Source: CAD feature listing. Evaluate the final solid. Frame: model axes, mm. A direction names the side the tool comes from. Coordinates: 2 decimals unless noted, no trailing zeros. Write each loop counter-clockwise with the first axis right and the second up, starting at its lowest first coordinate (ties: lowest second). Pieces come first, ordered by that corner, then holes. Notation, with made-up numbers: M -27,31.25 L 21,31.25 A22 ccw 21,43.25 Z; hole C 39,34.25 d8. An arc over 180 degrees is marked long. One line per item, written item: value. Start each with the question number.
Item 1: Cut plane A-A, the plane x = 0. Output: boundary loops of the cut face in (y, z), then the cut area to 3 significant figures.
Item 2: Cut plane C-C, the plane z = -10. Output: boundary loops of the cut face in (x, y).
Item 3: Cut plane D-D, the plane z = -14.25. Output: boundary loops of the cut face in (x, y), then the cut area to 3 significant figures.
Item 4: Set-up query: faces 1 (the flat face through (-2, -35, -5)), 2 (the flat face through (10, -28, 4)), 3 (the flat face through (5, 5, 7)). Return all of +Z, -Z, +X, -X, +Y, -Y with unobstructed straight access to the full face (end or side cutting, diameter ignored); none if empty.
Item 5: Cut plane B-B, the plane z = 5. Output: boundary loops of the cut face in (x, y).
Item 6: Mould query, pull axis X, two halves, no side actions, for faces 4 (the flat face through (-25, -48, -5)), 5 (the cylindrical face through (-15, -48, -8)), 6 (the flat face through (0, -48, -17)). Classes: released by +X, released by -X, zero draft, split by the parting line, or undercut.
Item 7: Ray query, L1, parallel to Z at x = 15, y = -46; L2, parallel to Y at x = -22.5, z = -15; L3, parallel to Z at x = -4.5, y = -25. Return the intervals inside material, ascending. Write a range as from..to.
Item 8: Pin query (flat end, axial travel): P1, Ø1.5, axis at x = -2.5, y = -27, coming from the -Z side; P2, Ø9, axis at y = -22.5, z = 2.5, coming from the +X side; P3, Ø1.5, axis at x = -18, z = -1, coming from the +Y side; P4, Ø12.5, axis at x = 0, y = 0, coming from the -Z side. Return the tip coordinate at first contact, or that it passes through.
```python
from build123d import *

# Parameters (mm, degrees)
BOSS_EXTRUDE1_DEPTH      = 8
CUT_EXTRUDE1_DEPTH       = 7
SKETCH2_W                = 50
SKETCH2_H                = 25
SKETCH2_R                = 2
BOSS_EXTRUDE2_DEPTH      = 5
BOSS_EXTRUDE3_DEPTH      = 2
BOSS_EXTRUDE3_DEPTH_BACK = 2


with BuildPart() as part:
    # Sketch1 → Boss-Extrude1 (new body)
    with BuildSketch(Plane.XY):
        with BuildLine():
            Line((10, -50), (10, -11.247333017))
            ThreePointArc((10, -11.247333017), (0, -15.05), (-10, -11.247333017))
            Line((-10, -11.247333017), (-10, -50))
            Line((-10, -50), (10, -50))
        make_face()
        with BuildLine():
            ThreePointArc((11.05, 0), (10.784305726, -2.408578419), (10, -4.701329599))
            Line((10, -4.701329599), (10, -11.247333017))
            ThreePointArc((10, -11.247333017), (13.72957574, -6.164515391), (15.05, 0))
            ThreePointArc((15.05, 0), (-6.164515391, 13.72957574), (-10, -11.247333017))
            Line((-10, -11.247333017), (-10, -4.701329599))
            ThreePointArc((-10, -4.701329599), (-2.408578419, 10.784305726), (11.05, 0))
        make_face()
        with BuildLine():
            Line((10, -11.247333017), (10, -4.701329599))
            ThreePointArc((10, -4.701329599), (0, -11.05), (-10, -4.701329599))
            Line((-10, -4.701329599), (-10, -11.247333017))
            ThreePointArc((-10, -11.247333017), (0, -15.05), (10, -11.247333017))
        make_face()
        with BuildLine():
            ThreePointArc((-6.847967297, 0), (0, 6.847967297), (6.847967297, 0))
            Line((6.847967297, 0), (10, 0))
            Line((10, 0), (10, -4.701329599))
            ThreePointArc((10, -4.701329599), (10.784305726, -2.408578419), (11.05, 0))
            ThreePointArc((11.05, 0), (-2.408578419, 10.784305726), (-10, -4.701329599))
            Line((-10, -4.701329599), (-10, 0))
            Line((-10, 0), (-6.847967297, 0))
        make_face()
        with BuildLine():
            Line((10, 0), (6.847967297, 0))
            ThreePointArc((6.847967297, 0), (0, -6.847967297), (-6.847967297, 0))
            Line((-6.847967297, 0), (-10, 0))
            Line((-10, 0), (-10, -4.701329599))
            ThreePointArc((-10, -4.701329599), (0, -11.05), (10, -4.701329599))
            Line((10, -4.701329599), (10, 0))
        make_face()
    extrude(amount=BOSS_EXTRUDE1_DEPTH)

    # Sketch1_3 → Cut-Extrude1 (cut)
    with BuildSketch(Plane.XY):
        with BuildLine():
            ThreePointArc((-6.847967297, 0), (0, 6.847967297), (6.847967297, 0))
            Line((6.847967297, 0), (10, 0))
            Line((10, 0), (10, -4.701329599))
            ThreePointArc((10, -4.701329599), (10.784305726, -2.408578419), (11.05, 0))
            ThreePointArc((11.05, 0), (-2.408578419, 10.784305726), (-10, -4.701329599))
            Line((-10, -4.701329599), (-10, 0))
            Line((-10, 0), (-6.847967297, 0))
        make_face()
        with BuildLine():
            Line((10, 0), (6.847967297, 0))
            ThreePointArc((6.847967297, 0), (0, -6.847967297), (-6.847967297, 0))
            Line((-6.847967297, 0), (-10, 0))
            Line((-10, 0), (-10, -4.701329599))
            ThreePointArc((-10, -4.701329599), (0, -11.05), (10, -4.701329599))
            Line((10, -4.701329599), (10, 0))
        make_face()
    extrude(amount=CUT_EXTRUDE1_DEPTH, mode=Mode.SUBTRACT)


with BuildPart() as cut_extrude1_kept_piece:
    # of the separate pieces the step leaves, the one the design keeps (cut_extrude1_pieces_kept)
    add(part.part.solids().sort_by_distance((-10, -11.247333017, 0))[0])

    # Sketch2 → Boss-Extrude2 (add)
    with BuildSketch(Plane.XZ.offset(50)):
        with Locations((0, -4.5)):
            Rectangle(SKETCH2_W, SKETCH2_H)
        with Locations((-15, -10)):
            Circle(SKETCH2_R, mode=Mode.SUBTRACT)
        with Locations((15, -10)):
            Circle(SKETCH2_R, mode=Mode.SUBTRACT)
    extrude(amount=-BOSS_EXTRUDE2_DEPTH)

    # Sketch5 → Boss-Extrude3 (add, two sides: drawn at the far end of the back side and taken through both)
    with BuildSketch(Plane(origin=(0, 0, 0), x_dir=(0, 0, -1), z_dir=(1, 0, 0)).offset(-BOSS_EXTRUDE3_DEPTH_BACK)):
        Polygon((0, -11.247333017), (17, -45), (0, -45), align=None)
    extrude(amount=BOSS_EXTRUDE3_DEPTH + BOSS_EXTRUDE3_DEPTH_BACK)


solid = cut_extrude1_kept_piece.part
```
From the geometry:
1. outline: M -50,-17 L -45,-17 L -11.25,0 L -11.05,0 L -11.05,7 L -6.85,7 L -6.85,8 L -50,8 Z; M 6.85,7 L 11.05,7 L 11.05,0 L 15.05,0 L 15.05,8 L 6.85,8 Z
1. area: 724 mm²
2. outline: M -25,-50 L -17,-50 L -17,-45 L -25,-45 Z; M -13,-50 L 13,-50 L 13,-45 L 2,-45 L 2,-31.1 L -2,-31.1 L -2,-45 L -13,-45 Z; M 17,-50 L 25,-50 L 25,-45 L 17,-45 Z
3. outline: M -25,-50 L 25,-50 L 25,-45 L 2,-45 L 2,-39.54 L -2,-39.54 L -2,-45 L -25,-45 Z
3. area: 272 mm²
4. face 1: -Z, -X, +Y
4. face 2: +Z, -Z, +X
4. face 3: -Z
5. outline: M -25,-50 L 25,-50 L 25,-45 L 10,-45 L 10,-11.25 A15.05 ccw long -10,-11.25 L -10,-45 L -25,-45 Z; hole C 0,0 d22.1
6. face 4: released by -X
6. face 5: undercut
6. face 6: zero draft
7. L1: z = -17..-12, -8..8
7. L2: y = -50..-45
7. L3: z = 0..8
8. P1: stops at z = -8.22
8. P2: stops at x = 10
8. P3: stops at y = -45
8. P4: passes through
